Part model, mm, in its own coordinate system. Face numbers are marked on the shaded views. A direction names the side the tool comes from. Round coordinates to 2 decimals unless told otherwise and drop trailing zeros. Write each loop counter-clockwise with the first axis right and the second up, starting at its lowest first coordinate (ties: lowest second). Pieces come first, ordered by that corner, then holes. Notation, with made-up numbers: (-36.5, 12) -> (0.5, 12) arc R20 cw to (0.5, 16) -> close; hole circle Ø7 at (49.25, 26.25). An arc over 180 degrees is marked (long way). Return JSON: item names as keys, results as strings. Group by question number.
(1) Saw through at B-B (z = 4.5). List the corners of the cut face in (x, y).
(2) Drill centre lines: L1, parallel to X at y = 3, z = 6.25; L2, parallel to Z at x = -0.25, y = 3.5; L3, parallel to Z at x = 0, y = 9.8. Where is each one in solid material? Low to high. Write a range as from..to.
(3) Saw through at C-C (y = 0). List the corners of the cut face in (x, z).
(4) Drop flat-ended pins along their axis: pin 1 Ø3 at (x, z) = (0.5, 3.5) entering from -Y; pin 2 Ø1.4 at (x, y) = (4.5, 0) entering from +Z; pin 3 Ø2 at (x, z) = (1.5, 6) entering from -Y; pin 4 Ø1.2 at (x, y) = (0, -1) entering from +Z. Give the stop position or say it passes through.
(5) Tool access for the marked faces 1, 2 and 3: list every direction of +Z, -Z, +X, -X, +Y, -Y with a clear straight run to the whole face (end or side of a thin tool).
(6) Saw through at A-A (y = 4). List the corners of the cut face in (x, z), plus the area to 3 significant figures.
(7) Saw through at D-D (x = 4.5). List the corners of the cut face in (y, z).
(8) Mould opens along X. For the marked faces 4, 5 and 6 say: +X half, -X half, draft (parallel to the pull), parting line (faces both ways), or undercut.
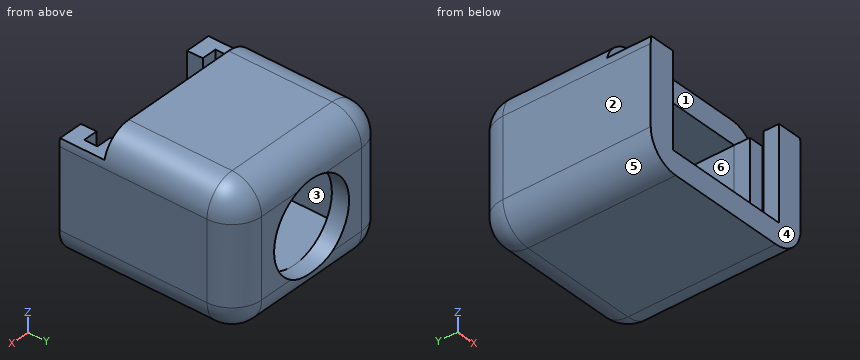
from build123d import *

# Parameters (mm, degrees)
F0_W         = 8.5
F0_H         = 7.834737435
F0_W_2       = 1.7211329822
F0_H_2       = 1.165262565
F0_W_3       = 1.7788670178
F1_DEPTH     = 0.9
F2_DEPTH     = 1.5
F3_DEPTH     = 7.8
F5_W         = 12
F5_H         = 9
F6_DEPTH     = 1.5
F7_R         = 3
F8_DEPTH     = 10.501
F9_T1_DEPTH  = 5.3
F9_T3_DEPTH  = 8
F9_T5_DEPTH  = 12
F9_T7_DEPTH  = 15
F9_S11_W     = 2
F9_S11_H     = 2
F9_T12_DEPTH = 2
F9_S17_W     = 2
F9_S17_H     = 2
F9_T18_DEPTH = 2
F9_S23_W     = 2
F9_S23_H     = 2
F9_T24_DEPTH = 2
F9_S29_W     = 2
F9_S29_H     = 2
F9_T30_DEPTH = 2


# Not quite as in the source:
# - a fillet or chamfer that OpenCascade refuses, or shapes differently, is made with other operations: its cross-section is extruded or revolved along the edge and cut away or added
# - a feature names something its author has since deleted; it is built from what else it names


with BuildPart() as f1:
    # F0 (on Top) → F1 (new body)
    with BuildSketch(Plane.XY):
        with Locations((-0.0288670178, 5.4173687175)):
            Rectangle(F0_W, F0_H)
        Polygon((-6, 1.5), (-6, -1.5), (-4.2211329822, -1.5), (-4.2413398946, -0.45), (-5.25, -0.45), (-5.25, 0.45), (-4.2586601054, 0.45), (-4.2788670178, 1.5), align=None)
        Polygon((4.2211329822, 1.5), (-4.2788670178, 1.5), (-4.2586601054, 0.45), (4.2413398946, 0.45), align=None)
        with Locations((-5.1394335089, 5.4173687175)):
            Rectangle(F0_W_2, F0_H)
        Polygon((4.2586601054, -0.45), (4.2788670178, -1.5), (6, -1.5), (6, 1.5), (4.2211329822, 1.5), (4.2413398946, 0.45), (5.25, 0.45), (5.25, -0.45), align=None)
        Polygon((-4.2413398946, -0.45), (-4.2211329822, -1.5), (4.2788670178, -1.5), (4.2586601054, -0.45), align=None)
        Polygon((-4.2586601054, 0.45), (-4.2413398946, -0.45), (4.2586601054, -0.45), (4.2413398946, 0.45), align=None)
        Polygon((-5.25, -0.45), (-4.2413398946, -0.45), (-4.2586601054, 0.45), (-5.25, 0.45), align=None)
        Polygon((4.2413398946, 0.45), (4.2586601054, -0.45), (5.25, -0.45), (5.25, 0.45), align=None)
        with Locations((-5.1394335089, 9.9173687175)):
            Rectangle(F0_W_2, F0_H_2)
        with Locations((-0.0288670178, 9.9173687175)):
            Rectangle(F0_W, F0_H_2)
        with Locations((5.1105664911, 9.9173687175)):
            Rectangle(F0_W_3, F0_H_2)
        with Locations((5.1105664911, 5.4173687175)):
            Rectangle(F0_W_3, F0_H)
    extrude(amount=F1_DEPTH)

    # F0 (on Top) → F2 (join)
    with BuildSketch(Plane.XY):
        Polygon((-4.2413398946, -0.45), (-4.2211329822, -1.5), (4.2788670178, -1.5), (4.2586601054, -0.45), align=None)
        Polygon((-6, 1.5), (-6, -1.5), (-4.2211329822, -1.5), (-4.2413398946, -0.45), (-5.25, -0.45), (-5.25, 0.45), (-4.2586601054, 0.45), (-4.2788670178, 1.5), align=None)
        Polygon((4.2586601054, -0.45), (4.2788670178, -1.5), (6, -1.5), (6, 1.5), (4.2211329822, 1.5), (4.2413398946, 0.45), (5.25, 0.45), (5.25, -0.45), align=None)
        Polygon((4.2211329822, 1.5), (-4.2788670178, 1.5), (-4.2586601054, 0.45), (4.2413398946, 0.45), align=None)
        with Locations((-5.1394335089, 5.4173687175)):
            Rectangle(F0_W_2, F0_H)
        with Locations((5.1105664911, 5.4173687175)):
            Rectangle(F0_W_3, F0_H)
        with Locations((-0.0288670178, 5.4173687175)):
            Rectangle(F0_W, F0_H)
        with Locations((-5.1394335089, 9.9173687175)):
            Rectangle(F0_W_2, F0_H_2)
        with Locations((-0.0288670178, 9.9173687175)):
            Rectangle(F0_W, F0_H_2)
        with Locations((5.1105664911, 9.9173687175)):
            Rectangle(F0_W_3, F0_H_2)
    extrude(amount=F2_DEPTH)

    # F0 (on Top) → F3 (join)
    with BuildSketch(Plane.XY):
        Polygon((-6, 1.5), (-6, -1.5), (-4.2211329822, -1.5), (-4.2413398946, -0.45), (-5.25, -0.45), (-5.25, 0.45), (-4.2586601054, 0.45), (-4.2788670178, 1.5), align=None)
        Polygon((4.2586601054, -0.45), (4.2788670178, -1.5), (6, -1.5), (6, 1.5), (4.2211329822, 1.5), (4.2413398946, 0.45), (5.25, 0.45), (5.25, -0.45), align=None)
        with Locations((-5.1394335089, 5.4173687175)):
            Rectangle(F0_W_2, F0_H)
        with Locations((5.1105664911, 5.4173687175)):
            Rectangle(F0_W_3, F0_H)
        with Locations((-5.1394335089, 9.9173687175)):
            Rectangle(F0_W_2, F0_H_2)
        with Locations((-0.0288670178, 9.9173687175)):
            Rectangle(F0_W, F0_H_2)
        with Locations((5.1105664911, 9.9173687175)):
            Rectangle(F0_W_3, F0_H_2)
    extrude(amount=F3_DEPTH)

    # F5 (on offset) → F6 (join)
    with BuildSketch(Plane.XY.offset(7.8)):
        with Locations((0, 6)):
            Rectangle(F5_W, F5_H)
    extrude(amount=F6_DEPTH)

    # F7 (on Front) → F8 (cut, through all)
    with BuildSketch(Plane.XZ):
        with Locations((0, 4.5)):
            Circle(F7_R)
    extrude(amount=-F8_DEPTH, mode=Mode.SUBTRACT)

    # F9: fillet of radius 2 on 8 edges, made by hand

    # F9_s2 → F9_t1 (cut)
    with BuildSketch(Plane.XY.offset(2)):
        with BuildLine():
            ThreePointArc((4, 10.5), (5.4142135624, 9.9142135624), (6, 8.5))
            Line((6, 8.5), (6, 10.5))
            Line((6, 10.5), (4, 10.5))
        make_face()
        with BuildLine():
            ThreePointArc((-4, 10.5), (-5.4142135624, 9.9142135624), (-6, 8.5))
            Line((-6, 8.5), (-6, 10.5))
            Line((-6, 10.5), (-4, 10.5))
        make_face()
    extrude(amount=F9_T1_DEPTH, mode=Mode.SUBTRACT)

    # F9_s4 → F9_t3 (cut)
    with BuildSketch(Plane.YZ.offset(-4)):
        with BuildLine():
            ThreePointArc((10.5, 7.3), (9.9142135624, 8.7142135624), (8.5, 9.3))
            Line((8.5, 9.3), (10.5, 9.3))
            Line((10.5, 9.3), (10.5, 7.3))
        make_face()
        with BuildLine():
            ThreePointArc((8.5, 0), (9.9142135624, 0.5857864376), (10.5, 2))
            Line((10.5, 2), (10.5, 0))
            Line((10.5, 0), (8.5, 0))
        make_face()
    extrude(amount=F9_T3_DEPTH, mode=Mode.SUBTRACT)

    # F9_s6 → F9_t5 (cut)
    with BuildSketch(Plane.XZ.offset(-8.5)):
        with BuildLine():
            ThreePointArc((4, 9.3), (5.4142135624, 8.7142135624), (6, 7.3))
            Line((6, 7.3), (6, 9.3))
            Line((6, 9.3), (4, 9.3))
        make_face()
        with BuildLine():
            ThreePointArc((-4, 9.3), (-5.4142135624, 8.7142135624), (-6, 7.3))
            Line((-6, 7.3), (-6, 9.3))
            Line((-6, 9.3), (-4, 9.3))
        make_face()
    extrude(amount=F9_T5_DEPTH, mode=Mode.SUBTRACT)

    # F9_s8 → F9_t7 (cut)
    with BuildSketch(Plane.XZ.offset(-8.5)):
        with BuildLine():
            ThreePointArc((4, 0), (5.4142135624, 0.5857864376), (6, 2))
            Line((6, 2), (6, 0))
            Line((6, 0), (4, 0))
        make_face()
        with BuildLine():
            ThreePointArc((-4, 0), (-5.4142135624, 0.5857864376), (-6, 2))
            Line((-6, 2), (-6, 0))
            Line((-6, 0), (-4, 0))
        make_face()
    extrude(amount=F9_T7_DEPTH, mode=Mode.SUBTRACT)


with BuildPart() as f9_tool10:
    # F9_s11 → F9_t12 (new body)
    with BuildSketch(Plane.XY.offset(2)):
        with Locations((5, 9.5)):
            Rectangle(F9_S11_W, F9_S11_H)
    extrude(amount=-F9_T12_DEPTH)

    # F9_s13 → F9_t14 (revolve, cut)
    with BuildSketch(Plane(origin=(4, 8.5, 2), x_dir=(-0.7071067812, -0.7071067812, 0), z_dir=(0.7071067812, -0.7071067812, 0))):
        with BuildLine():
            ThreePointArc((0, -2), (2, 0), (0, 2))
            Line((0, 2), (0, -2))
        make_face()
    revolve(axis=Axis((4, 8.5, 2), (0, 0, -1)), mode=Mode.SUBTRACT)


with BuildPart() as f1_1:
    add(f1.part)

    # F9_t9: cut F9_tool10
    add(f9_tool10.part, mode=Mode.SUBTRACT)


with BuildPart() as f9_tool16:
    # F9_s17 → F9_t18 (new body)
    with BuildSketch(Plane.XY.offset(7.3)):
        with Locations((5, 9.5)):
            Rectangle(F9_S17_W, F9_S17_H)
    extrude(amount=F9_T18_DEPTH)

    # F9_s19 → F9_t20 (revolve, cut)
    with BuildSketch(Plane(origin=(4, 8.5, 7.3), x_dir=(-0.7071067812, -0.7071067812, 0), z_dir=(-0.7071067812, 0.7071067812, 0))):
        with BuildLine():
            ThreePointArc((0, -2), (2, 0), (0, 2))
            Line((0, 2), (0, -2))
        make_face()
    revolve(axis=Axis((4, 8.5, 7.3), (0, 0, 1)), mode=Mode.SUBTRACT)


with BuildPart() as f1_2:
    add(f1_1.part)

    # F9_t15: cut F9_tool16
    add(f9_tool16.part, mode=Mode.SUBTRACT)


with BuildPart() as f9_tool22:
    # F9_s23 → F9_t24 (new body)
    with BuildSketch(Plane.YZ.offset(-4)):
        with Locations((9.5, 8.3)):
            Rectangle(F9_S23_W, F9_S23_H)
    extrude(amount=-F9_T24_DEPTH)

    # F9_s25 → F9_t26 (revolve, cut)
    with BuildSketch(Plane(origin=(-4, 8.5, 7.3), x_dir=(0, -0.7071067812, -0.7071067812), z_dir=(0, 0.7071067812, -0.7071067812))):
        with BuildLine():
            ThreePointArc((0, -2), (2, 0), (0, 2))
            Line((0, 2), (0, -2))
        make_face()
    revolve(axis=Axis((-4, 8.5, 7.3), (-1, 0, 0)), mode=Mode.SUBTRACT)


with BuildPart() as f1_3:
    add(f1_2.part)

    # F9_t21: cut F9_tool22
    add(f9_tool22.part, mode=Mode.SUBTRACT)


with BuildPart() as f9_tool28:
    # F9_s29 → F9_t30 (new body)
    with BuildSketch(Plane.YZ.offset(-4)):
        with Locations((9.5, 1)):
            Rectangle(F9_S29_W, F9_S29_H)
    extrude(amount=-F9_T30_DEPTH)

    # F9_s31 → F9_t32 (revolve, cut)
    with BuildSketch(Plane(origin=(-4, 8.5, 2), x_dir=(0, -0.7071067812, 0.7071067812), z_dir=(0, -0.7071067812, -0.7071067812))):
        with BuildLine():
            ThreePointArc((0, -2), (2, 0), (0, 2))
            Line((0, 2), (0, -2))
        make_face()
    revolve(axis=Axis((-4, 8.5, 2), (-1, 0, 0)), mode=Mode.SUBTRACT)


with BuildPart() as f1_4:
    add(f1_3.part)

    # F9_t27: cut F9_tool28
    add(f9_tool28.part, mode=Mode.SUBTRACT)


solid = f1_4.part
Computed values:
{
 "1": {"outline": "(-6, -1.5) -> (-4.22, -1.5) -> (-4.24, -0.45) -> (-5.25, -0.45) -> (-5.25, 0.45) -> (-4.26, 0.45) -> (-4.28, 1.5) -> (-4.28, 9.33) -> (-3, 9.33) -> (-3, 10.5) -> (-4, 10.5) arc R2 ccw to (-6, 8.5) -> close; (3, 9.33) -> (4.22, 9.33) -> (4.22, 1.5) -> (4.24, 0.45) -> (5.25, 0.45) -> (5.25, -0.45) -> (4.26, -0.45) -> (4.28, -1.5) -> (6, -1.5) -> (6, 8.5) arc R2 ccw to (4, 10.5) -> (3, 10.5) -> close"},
 "2": {"L1": "-6..-4.28, 4.22..6", "L2": "0..1.5, 7.8..9.3", "L3": "0.48..1.5, 7.5..8.82"},
 "3": {"outline": "(-6, 2) arc R2 ccw to (-4, 0) -> (4, 0) arc R2 ccw to (6, 2) -> (6, 7.3) arc R2 ccw to (5.94, 7.8) -> (5.25, 7.8) -> (5.25, 0.9) -> (-5.25, 0.9) -> (-5.25, 7.8) -> (-5.94, 7.8) arc R2 ccw to (-6, 7.3) -> close"},
 "4": {"pin 1": "through", "pin 2": "z = 7.8", "pin 3": "y = 9.33", "pin 4": "z = 1.5"},
 "5": {"face 1": "+Z, +X, -X, -Y", "face 2": "+Z, -Z, -X, +Y, -Y", "face 3": "none"},
 "6": {"outline": "(-6, 2) arc R2 ccw to (-4, 0) -> (4, 0) arc R2 ccw to (6, 2) -> (6, 7.3) arc R2 ccw to (4, 9.3) -> (-4, 9.3) arc R2 ccw to (-6, 7.3) -> close; hole (-4.28, 1.5) -> (4.22, 1.5) -> (4.22, 7.8) -> (-4.28, 7.8) -> close", "area": "54.6 mm2"},
 "7": {"outline": "(-1.5, 0.06) -> (8.5, 0.06) arc R1.94 ccw to (10.44, 2) -> (10.44, 7.3) arc R1.94 ccw to (8.5, 9.24) -> (1.5, 9.24) -> (1.5, 7.8) -> (0.45, 7.8) -> (0.45, 0.9) -> (-0.45, 0.9) -> (-0.45, 7.8) -> (-1.5, 7.8) -> close"},
 "8": {"face 4": "draft", "face 5": "-X half", "face 6": "undercut"}
}
